Input: part model. Units: mm. Frame: model coordinates. A direction names the side the tool comes from. Coordinates: 2 decimals unless noted, no trailing zeros. Write each loop counter-clockwise with the first axis right and the second up, starting at its lowest first coordinate (ties: lowest second). Pieces come first, ordered by that corner, then holes. Notation, with made-up numbers: M 60.5,53 L 92.5,53 A23 cw 92.5,91 Z; hole C 64.25,16 d3. An arc over 180 degrees is marked long. Write each question's results on one line, items separated by ' | '. Start each with the question number.
1. Section query C-C, the plane x = -59. Output: boundary loops of the cut face in (y, z).
2. Section query B-B, the plane y = 148. Output: boundary loops of the cut face in (x, z).
3. Pull-direction query (X, two-part tool) for faces 1 (the flat face through (28.571, 236.384, 385.433)), 2 (the flat face through (172.25, -111.41, 406.82)), 3 (the flat face through (-127.763, 80.764, 356.3)); classes: +X half, -X half, draft (parallel to the pull), parting line (faces both ways), or undercut.
4. First-contact query: pin 1 (6.5 mm diameter, centred on y = -68, z = 481.5, fed in from -X); pin 2 (5 mm diameter, centred on x = -98.5, z = 358.5, fed in from +Y); pin 3 (16.5 mm diameter, centred on y = -74.5, z = 480.5, fed in from +X); pin 4 (8 mm diameter, centred on x = -46, y = 58.5, fed in from -Z). Flat tips, straight axial feed; report the tip coordinate or a pass-through.
5. Section query A-A, the plane z = 570.5. Output: boundary loops of the cut face in (x, y), and give its area (3 significant figures).
6. Section query D-D, the plane z = 216. Output: boundary loops of the cut face in (x, y).
7. Set-up query: faces 4 (the flat face through (-202.57, -143.96, 218.32)), 5 (the flat face through (-108.777, -71, 481)), 6 (the flat face through (0, -71, 481)), 7 (the flat face through (38, -29, 0)). Return all of +Z, -Z, +X, -X, +Y, -Y with unobstructed straight access to the full face (end or side cutting, diameter ignored); none if empty.
8. Ray query, probe 1 along X at (y, z) = (-51.5, 588.5); probe 2 along Y at (x, z) = (28, 223.5); probe 3 along X at (y, z) = (-111, 357). Return the intervals inside material, ascending.
```python
from build123d import *

# Parameters (mm, degrees)
F6_DEPTH  = 50
F8_DEPTH  = 50
F11_DEPTH = 10
F9_W      = 108.7769791484
F9_H      = 37.0438992977
F12_DEPTH = 12.7


with BuildPart() as f4:
    # F0 (on Top) → F4 section 0
    with BuildSketch(Plane.XY, mode=Mode.PRIVATE) as f4_s0:
        Polygon((-433.0127018922, -250), (433.0127018922, -250), (0, 500), align=None)
    loft([f4_s0.sketch, Vertex(0, 0, 900)])

    # F5 (on face) → F6 (cut)
    with BuildSketch(Plane(origin=(0, -232.0916905444, 64.4699140401), x_dir=(1, 0, 0), z_dir=(0, -0.9635179096, 0.2676438638))):
        Polygon((339.7423923016, 0), (0, 734.6025705338), (-340.5417487738, 0), align=None)
    extrude(amount=-F6_DEPTH, mode=Mode.SUBTRACT)

    # F7 (on face) → F8 (cut)
    with BuildSketch(Plane(origin=(200.9973000187, 116.0458452722, 64.4699140401), x_dir=(-0.458738865, 0.8763037769, -0.1471405596), z_dir=(0.8344309867, 0.4817589548, 0.2676438638))):
        Polygon((291.1387085915, 69.377720356), (-116.6230589151, 700.2393603325), (-308.3382844925, -33.8495075703), align=None)
    extrude(amount=-F8_DEPTH, mode=Mode.SUBTRACT)

    # F10 (on face) → F11 (join)
    with BuildSketch(Plane(origin=(0, -232.0916905444, 64.4699140401), x_dir=(1, 0, 0), z_dir=(0, -0.9635179096, 0.2676438638))):
        with BuildLine():
            add(Edge.make_bspline(
                [(40.1289761066, -39.7394858301), (40.1289761066, -9.8174087107), (-20.0644880533, -24.7784472704), (-80.2579522133, -39.7394858301), (-20.0644880533, -54.7005243897), (40.1289761066, -69.6615629494), (40.1289761066, -39.7394858301)],
                knots=[0, 0, 0, 2.0943951024, 2.0943951024, 4.1887902048, 4.1887902048, 6.2831853072, 6.2831853072, 6.2831853072], degree=2, weights=[1, 0.5, 1, 0.5, 1, 0.5, 1]))
        make_face()
    extrude(amount=F11_DEPTH)

    # F9 (on face) → F12 (join)
    with BuildSketch(Plane(origin=(0, -183.9157950629, 51.0877208508), x_dir=(1, 0, 0), z_dir=(0, -0.9635179096, 0.2676438638))):
        Polygon((-164.8651063442, 258.7849199772), (-241.3489073515, 82.3854953051), (-44.1906489432, 84.1495096684), (-44.1906489432, 258.7849199772), align=None)
        Polygon((100.2787798643, 258.7849199772), (0, 258.7849199772), (0, 82.3854953051), (227.7518063784, 82.3854953051), align=None)
        Polygon((-110.4766204953, 389.3205523491), (-108.7769791484, 350.5126535892), (73.084525764, 350.5126535892), (73.084525764, 389.3205523491), align=None)
        with Locations((-54.3884895742, 444.886341691)):
            Rectangle(F9_W, F9_H)
        Polygon((67.9856017232, 458.1163227558), (33.9928083122, 461.6443216801), (33.9928083122, 426.3643920422), (67.9856017232, 426.3643920422), align=None)
    extrude(amount=F12_DEPTH)


solid = f4.part
```
Answer:
1) outline: M -250,0 L 397.81,0 L -34.06,777.37 L -69.54,649.64 L -21.37,636.26 L -59.89,497.59 L -72.12,500.99 L -82.04,465.3 L -69.8,461.9 L -79.72,426.21 L -91.95,429.6 L -102.34,392.21 L -90.1,388.81 L -114.65,300.43 L -126.89,303.83 L -173.67,135.44 L -161.43,132.04 L -183.92,51.09 L -232.09,64.47 Z
2) outline: M -203.23,0 L 203.23,0 L 176.47,83.41 L 120.7,70.49 L 1.4,442.43 L 42.74,500.35 L 0,633.6 Z
3) face 1: +X half | face 2: undercut | face 3: -X half
4) pin 1: x = -175.64 | pin 2: y = 134.77 | pin 3: x = 183.02 | pin 4: z = 0
5) outline: M -158.53,-91.53 L -97.08,-91.53 L -90.64,-39.63 L 68.65,-39.63 L 0.31,78.74 L 42.14,110.06 L 0,183.06 Z; M 91.05,-44.7 L 96.85,-91.53 L 158.53,-91.53 L 123.42,-30.71 Z | area: 25,900 mm^2
6) outline: M -329.09,-190 L -267.64,-190 L -261.2,-138.11 L -202.86,-138.11 L -204.39,-151.29 L -44.19,-151.29 L -44.19,-138.11 L 0,-138.11 L 0,-151.29 L 166.15,-151.29 L 163.6,-138.11 L 239.21,-138.11 L 3.32,270.46 L 45.16,301.78 L 0,380 Z; M 245.34,-138.11 L 260.59,-138.11 L 267.01,-190 L 329.09,-190 L 288.38,-119.49 Z
7) face 4: none | face 5: -Y | face 6: +Z, -Y | face 7: -Z, +X, -X, +Y, -Y
8) probe 1: -129.65 to -84.07, 83.87 to 129.65 | probe 2: -149.2 to 223.55, 284.93 to 327.34 | probe 3: -238.25 to -194.86, 194.4 to 238.25
